Drawing for the job (mm, zero at the part's lowest x, y, z). A direction names the side the tool comes from. Round coordinates to 2 decimals unless told otherwise and drop trailing zeros. Write each loop counter-clockwise with the first axis right and the second up, starting at its lowest first coordinate (ties: lowest second). Pieces come first, ordered by that corner, then holes. Notation, with made-up numbers: M 13.5,-5.75 L 35.5,-5.75 A21 cw 35.5,14.25 Z; hole C 54,64.25 d7. An arc over 180 degrees is marked long. Use a Markdown table: item, result. Add a question column.
1) Which spindle directions (+Z, -Z, +X, -X, +Y, -Y) get a long thin tool onto all of the face, cutting with end or side? Do the marked faces 1 and 2. Say none if no direction does.
2) Slice it at C-C on z = 7.5. Write the cut outline in (x, y) (1 decimal).
3) Slice it at B-B on y = 47.5. Write the cut outline in (x, z) (1 decimal).
4) Slice it at A-A on x = 50.8. Write the cut outline in (y, z) (1 decimal).
5) Slice it at D-D on x = 31.75. Write the cut outline in (y, z) (1 decimal).
6) Wall check: probe 1 along Y at (x, z) = (12.7, 1.1) (1 decimal); probe 2 along Z at (x, y) = (38, 29) (1 decimal). Give the ranges that are in metal, low to high.
7) Drop flat-ended pins along their axis: P1, Ø6, axis at x = 30.5, y = 39, coming from the +Z side (1 decimal); P2, Ø24, axis at x = 43, z = 16.5, coming from the +Y side (1 decimal). Give the stop position or say it passes through.
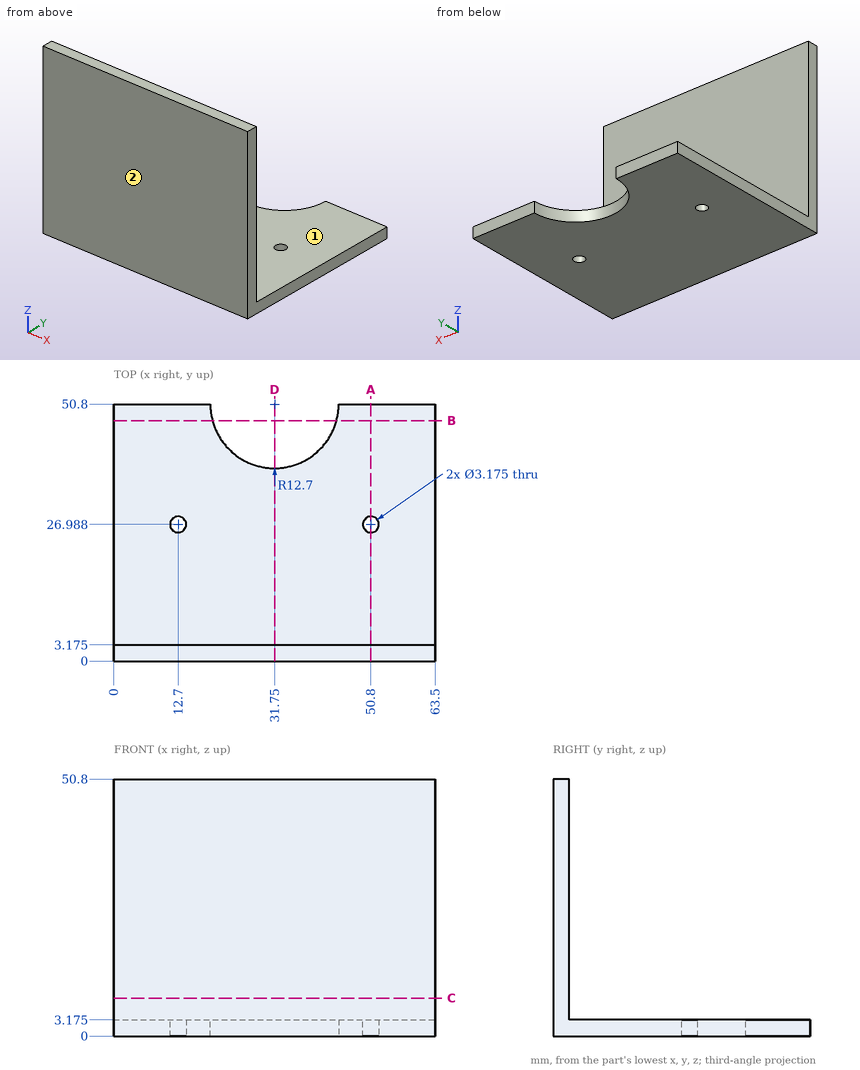
Entries:
| question | item | result |
|---|---|---|
| 1 | face 1 | +Z, +X, -X, +Y |
| 1 | face 2 | +Z, -Z, +X, -X, -Y |
| 2 | outline | M 0,0 L 63.5,0 L 63.5,3.2 L 0,3.2 Z |
| 3 | outline | M 0,0 L 19.5,0 L 19.5,3.2 L 0,3.2 Z; M 44,0 L 63.5,0 L 63.5,3.2 L 44,3.2 Z |
| 4 | outline | M 0,0 L 25.4,0 L 25.4,3.2 L 3.2,3.2 L 3.2,50.8 L 0,50.8 Z; M 28.6,0 L 50.8,0 L 50.8,3.2 L 28.6,3.2 Z |
| 5 | outline | M 0,0 L 38.1,0 L 38.1,3.2 L 3.2,3.2 L 3.2,50.8 L 0,50.8 Z |
| 6 | probe 1 | y = 0 to 25.4, 28.6 to 50.8 |
| 6 | probe 2 | z = 0 to 3.2 |
| 7 | P1 | stops at z = 3.2 |
| 7 | P2 | stops at y = 3.2 |
